Here's how the part is built. I have some questions about the finished solid (model axes, mm). A direction names the side the tool comes from. Round coordinates to 2 decimals unless told otherwise and drop trailing zeros. Loops run counter-clockwise (first coordinate to the right, second up) from the corner with the lowest first, then second, coordinate; pieces in that order, holes last. Notation, with made-up numbers: M 39.25,43 L 49.25,43 A35 ccw 49.25,77 Z; hole C 65.25,16 d2. An arc over 180 degrees is marked long. Put each result on its own line as item: value. Start each with the question number.
```python
from build123d import *

# Parameters (mm, degrees)
F0_W     = 14
F0_H     = 14
F1_DEPTH = 2
F2_R     = 6
F2_R_2   = 3.5
F3_DEPTH = 5
F4_SIZE2 = 3
F4_SIZE  = 1
F9_DEPTH = 2
F10_R    = 2


with BuildPart() as f1:
    # F0 (on Top) → F1 (new body)
    with BuildSketch(Plane.XY):
        with Locations((-7, 7)):
            Rectangle(F0_W, F0_H)
    extrude(amount=F1_DEPTH)

    # F2 (on face) → F3 (join)
    with BuildSketch(Plane.XY.offset(2)):
        with Locations((-7, 7)):
            Circle(F2_R)
        with Locations((-7, 7)):
            Circle(F2_R_2, mode=Mode.SUBTRACT)
    extrude(amount=F3_DEPTH)

    # F4
    f4_edges = [f1.edges().sort_by_distance(p)[0] for p in [
        (-13, 7, 7),
    ]]
    f4_side = f1.faces().sort_by_distance((-12.830294, 7, 7))[0]
    chamfer(f4_edges, length=F4_SIZE, length2=F4_SIZE2, reference=f4_side)


with BuildPart() as f1_1:
    # F5: moved
    add(f1.part.moved(Location((7, 0, 0))))

    # F6 (on Right) → F7 (revolve, cut)
    with BuildSketch(Plane.YZ):
        Polygon((13, 2), (13, 4), (12.5, 2), align=None)
    revolve(axis=Axis((0, 7, 22.9139531255), (0, 0, 1)), mode=Mode.SUBTRACT)

    # F8 (on face) → F9 (cut, through all)
    with BuildSketch(Plane.XY.offset(2)):
        with BuildLine():
            Line((1, 3.6458980338), (1, 10.3541019662))
            ThreePointArc((1, 10.3541019662), (0, 10.5), (-1, 10.3541019662))
            Line((-1, 10.3541019662), (-1, 3.6458980338))
            ThreePointArc((-1, 3.6458980338), (0, 3.5), (1, 3.6458980338))
        make_face()
    extrude(amount=-F9_DEPTH, mode=Mode.SUBTRACT)

    # F10
    f10_edges = [f1_1.edges().sort_by_distance(p)[0] for p in [
        (7, 0, 1),
        (7, 14, 1),
        (-7, 14, 1),
        (-7, 0, 1),
    ]]
    fillet(f10_edges, radius=F10_R)


solid = f1_1.part
```
1) I'm going to push flat-ended pins straight in: P1, Ø2, axis at y = 8.5, z = 6, coming from the +X side; P2, Ø4, axis at y = 6.5, z = 5.5, coming from the +X side; P3, Ø4, axis at x = 0, y = 7, coming from the +Z side. Where does each tip first touch, or does it pass through?
2) On a 3-axis mill with a long thin cutter (end or side, diameter ignored), from which of +Z, -Z, +X, -X, +Y, -Y can I reach the whole of each face in a straight line? I mean faces 1 (the face through (-5, 10, 2)), 2 (the face through (0, 14, 1)), 3 (the face through (2, 7, 2)), 4 (the face through (-1, 7, 1)). Say none if no direction works.
3) If I drill on probe 1 along X at (y, z) = (7, 4); probe 2 along Z at (x, y) = (-6, 4.75); probe 3 along Y at (x, z) = (1.5, 5.5), over which ranges is the centre line in solid material (lowest first)? Write a range as from..to.
4) Suppose I cut it at B-B (y = 7). Write out the boundary of the cut face in (x, z).
5) Suppose I cut it at C-C (z = 3). Write out the boundary of the cut face in (x, y).
6) Suppose I cut it at D-D (z = 6.25). Write out the boundary of the cut face in (x, y), plus the area to 3 significant figures.
7) If we mould it in two halves opening along Y, with no side actions, what happens to faces 5 (the face through (-7, 7, 1)), 6 (the face through (-2, 7, 2)), 7 (the face through (6.4, 13.43, 1.01))? For each: pulls with the +Y half, pulls with the -Y half, needs draft (parallel to the pull), parting line crosses it, or undercut.
8) Suppose I cut it at A-A (x = 0). Write out the boundary of the cut face in (y, z), plus the area to 3 significant figures.
Results are:
1. P1: x = 5.53
1. P2: x = 6
1. P3: z = 2
2. face 1: none
2. face 2: +Z, -Z, +X, -X, +Y
2. face 3: +Z
2. face 4: +Z, -Z
3. probe 1: -6..-3.5, 3.5..6
3. probe 2: 0..2
3. probe 3: 1.71..3.84, 10.16..12.29
4. outline: M -7,0 L -1,0 L -1,2 L -3.5,2 L -3.5,7 L -5,7 L -6,4 L -5.5,2 L -7,2 Z; M 1,0 L 7,0 L 7,2 L 5.5,2 L 6,4 L 5,7 L 3.5,7 L 3.5,2 L 1,2 Z
5. outline: C 0,7 d11.5; hole C 0,7 d7
6. outline: C 0,7 d10.5; hole C 0,7 d7
6. area: 48.1 mm²
7. face 5: needs draft
7. face 6: undercut
7. face 7: pulls with the +Y half
8. outline: M 0,0 L 3.5,0 L 3.5,7 L 2,7 L 1,4 L 1.5,2 L 0,2 Z; M 10.5,0 L 14,0 L 14,2 L 12.5,2 L 13,4 L 12,7 L 10.5,7 Z
8. area: 35.0 mm²
